Read the model definition and answer for the solid it produces. Units are mm, in the model's axes. A direction names the side the tool comes from. Round coordinates to 2 decimals unless told otherwise and drop trailing zeros. Order: outer loops, then holes, each group sorted by start corner. A loop starts at its lowest first (then second) coordinate and runs counter-clockwise, first axis right, second up. Notation, with made-up numbers: M -31,10 L 27,10 A23 cw 27,34 Z; hole C -19.5,-29.5 d4. An arc over 180 degrees is marked long. Answer as CSV lines item,"result".
```python
from build123d import *

# Parameters (mm, degrees)
F2_R          = 0.25
F3_R          = 2.25
F4_DEPTH      = 25
F5_R          = 1.65
F6_DEPTH      = 25
F6_DEPTH_BACK = 25
F7_R          = 1.75
F8_DEPTH      = 25
F8_DEPTH_BACK = 25


with BuildPart() as f1:
    # F0 (on Right) → F1 (revolve)
    with BuildSketch(Plane.YZ):
        Polygon((0, 29), (0, 8.25), (17.5, 8.25), (17.5, 13.25), (5.5, 13.25), (5.5, 29), align=None)
    revolve(axis=Axis((0, 5.341735, 0), (0, 1, 0)))

    # F2
    f2_edges = [f1.edges().sort_by_distance(p)[0] for p in [
        (0, 5.5, -13.25),
    ]]
    fillet(f2_edges, radius=F2_R)

    # F3 (on face) → F4 (cut)
    with BuildSketch(Plane(origin=(0, 5.5, 0), x_dir=(-1, 0, 0), z_dir=(0, 1, 0))):
        with Locations((-15.5, 15.5)):
            Circle(F3_R)
        with Locations((15.5, 15.5)):
            Circle(F3_R)
        with Locations((-15.5, -15.5)):
            Circle(F3_R)
        with Locations((15.5, -15.5)):
            Circle(F3_R)
    extrude(amount=-F4_DEPTH, mode=Mode.SUBTRACT)

    # F5 (on Top) → F6 (cut, two sides)
    with BuildSketch(Plane.XY) as f6_sk:
        with Locations((0, 11.5)):
            Circle(F5_R)
    extrude(amount=F6_DEPTH, mode=Mode.SUBTRACT)
    extrude(f6_sk.sketch, amount=-F6_DEPTH_BACK, mode=Mode.SUBTRACT)

    # F7 (on Right) → F8 (cut, two sides)
    with BuildSketch(Plane.YZ) as f8_sk:
        with Locations((11.5, 0)):
            Circle(F7_R)
    extrude(amount=F8_DEPTH, mode=Mode.SUBTRACT)
    extrude(f8_sk.sketch, amount=-F8_DEPTH_BACK, mode=Mode.SUBTRACT)


solid = f1.part
```
Item 1: A cutting plane is placed at D-D, the plane z = -15.5. Determine the outline of the cut face in (x, y).
Ans:
outline,"M -24.51,0 L -17.75,0 L -17.75,5.5 L -24.51,5.5 Z; M -13.25,0 L 13.25,0 L 13.25,5.5 L -13.25,5.5 Z; M 17.75,0 L 24.51,0 L 24.51,5.5 L 17.75,5.5 Z"
Item 2: A cutting plane is placed at A-A, the plane z = 0. Determine the outline of the cut face in (x, y), and give its area (3 significant figures).
Ans:
outline,"M -29,0 L -8.25,0 L -8.25,9.75 L -13.25,9.75 L -13.25,5.75 A0.25 cw -13.5,5.5 L -29,5.5 Z; M -13.25,13.25 L -8.25,13.25 L -8.25,17.5 L -13.25,17.5 Z; M 8.25,0 L 29,0 L 29,5.5 L 13.5,5.5 A0.25 cw 13.25,5.75 L 13.25,9.75 L 8.25,9.75 Z; M 8.25,13.25 L 13.25,13.25 L 13.25,17.5 L 8.25,17.5 Z"
area,"313 mm2"
Item 3: Flat-ended cylindrical pins translate along their axes: pin 1 (2 mm diameter, centred on x = 0, y = 11.5, fed in from +Z); pin 2 (8 mm diameter, centred on y = 7.5, z = -9.5, fed in from +X); pin 3 (4 mm diameter, centred on x = -18, z = -8, fed in from +Y); pin 4 (4 mm diameter, centred on x = 6, y = 5, fed in from -Z). Find the tip coordinate at first contact, or state that the pin passes through.
Ans:
pin 1,"through"
pin 2,"x = 28.36"
pin 3,"y = 5.5"
pin 4,"z = -28.72"
Item 4: Determine the mould class of faces 3 (the face through (-10.621, 13.169, 0.526)), 4 (the face through (-25.73, 2.71, 13.38)), 5 (the face through (10.621, 13.169, 0.526)), 6 (the face through (-6, 5.5, -12.5)) for opening direction Y: +Y half, -Y half, draft (parallel to the pull), parting line (faces both ways), or undercut.
Ans:
face 3,"undercut"
face 4,"draft"
face 5,"undercut"
face 6,"+Y half"
Item 5: A cutting plane is placed at C-C, the plane y = 12.25. Determine the outline of the cut face in (x, z).
Ans:
outline,"M -13.16,-1.58 A13.25 ccw -1.47,-13.17 L -1.47,-8.12 A8.25 cw -8.1,-1.58 Z; M -13.16,1.58 L -8.1,1.58 A8.25 cw -1.47,8.12 L -1.47,13.17 A13.25 ccw Z; M 1.47,-13.17 A13.25 ccw 13.16,-1.58 L 8.1,-1.58 A8.25 cw 1.47,-8.12 Z; M 1.47,8.12 A8.25 cw 8.1,1.58 L 13.16,1.58 A13.25 ccw 1.47,13.17 Z"
Item 6: A tool of negligible diameter and unlimited length cuts with its end or side. For faces 1 (the face through (-16.538, 2.788, 13.504)), 2 (the face through (-5.07, 11.54, 12.24)), from which of +Z, -Z, +X, -X, +Y, -Y can it reach the whole face along a straight path? Write none if from no direction.
Ans:
face 1,"+Y, -Y"
face 2,"+Y"
Item 7: A cutting plane is placed at B-B, the plane x = 0. Determine the outline of the cut face in (y, z).
Ans:
outline,"M 0,-29 L 5.5,-29 L 5.5,-13.5 A0.25 cw 5.75,-13.25 L 9.85,-13.25 L 9.85,-8.25 L 0,-8.25 Z; M 0,8.25 L 9.85,8.25 L 9.85,13.25 L 5.75,13.25 A0.25 cw 5.5,13.5 L 5.5,29 L 0,29 Z; M 13.15,-13.25 L 17.5,-13.25 L 17.5,-8.25 L 13.15,-8.25 Z; M 13.15,8.25 L 17.5,8.25 L 17.5,13.25 L 13.15,13.25 Z"
Item 8: Find the intervals of material crossed by probe 1 along Y at (x, z) = (-12, 0); probe 2 along Z at (x, y) = (15.5, 2.4); probe 3 along Z at (x, y) = (-16, 2.25), in increasing order. Write a range as [from, to].
Ans:
probe 1,"[0, 9.75], [13.25, 17.5]"
probe 2,"[-24.51, -17.75], [-13.25, 13.25], [17.75, 24.51]"
probe 3,"[-24.19, -17.69], [-13.31, 13.31], [17.69, 24.19]"
